Part model, mm, in its own coordinate system. Face numbers are marked on the shaded views. A direction names the side the tool comes from. Round coordinates to 2 decimals unless told otherwise and drop trailing zeros. Loops run counter-clockwise (first coordinate to the right, second up) from the corner with the lowest first, then second, coordinate; pieces in that order, holes last.
from build123d import *

# Parameters (mm, degrees)
BOSS_EXTRUDE1_DEPTH = 58
SKETCH2_R           = 6
BOSS_EXTRUDE2_DEPTH = 1
SKETCH3_R           = 4
BOSS_EXTRUDE3_DEPTH = 5
CUT_EXTRUDE1_DEPTH  = 3
FILLET1_R           = 0.5


with BuildPart() as part:
    # Sketch1 → Boss-Extrude1 (new body)
    with BuildSketch(Plane(origin=(0, 0, 0), x_dir=(1, 0, 0), z_dir=(0, 1, 0))):
        Polygon((0, 50), (0, 0), (50, 0), (50, 8), (30, 8), (8, 30), (8, 50), align=None)
        Polygon((5, 25.928932188), (25.928932188, 5), (5, 5), align=None, mode=Mode.SUBTRACT)
    extrude(amount=BOSS_EXTRUDE1_DEPTH)

    # Sketch2 → Boss-Extrude2 (add)
    with BuildSketch(Plane(origin=(8, 0, 0), x_dir=(0, 0, -1), z_dir=(1, 0, 0))):
        with Locations((40, 29)):
            Circle(SKETCH2_R)
    extrude(amount=BOSS_EXTRUDE2_DEPTH)

    # Sketch3 → Boss-Extrude3 (add)
    with BuildSketch(Plane(origin=(9, 0, 0), x_dir=(0, 0, -1), z_dir=(1, 0, 0))):
        with Locations((40, 29)):
            Circle(SKETCH3_R)
    extrude(amount=BOSS_EXTRUDE3_DEPTH)

    # Sketch4 → Cut-Extrude1 (cut)
    with BuildSketch(Plane(origin=(14, 0, 0), x_dir=(0, 0, -1), z_dir=(1, 0, 0))):
        Polygon((40, 26.401923789), (42.25, 27.700961894), (42.25, 30.299038106), (40, 31.598076211), (37.75, 30.299038106), (37.75, 27.700961894), align=None)
    extrude(amount=-CUT_EXTRUDE1_DEPTH, mode=Mode.SUBTRACT)

    # Fillet1
    fillet1_edges = [part.edges().sort_by_distance(p)[0] for p in [
        (14, 29, -36),
    ]]
    fillet(fillet1_edges, radius=FILLET1_R)


solid = part.part
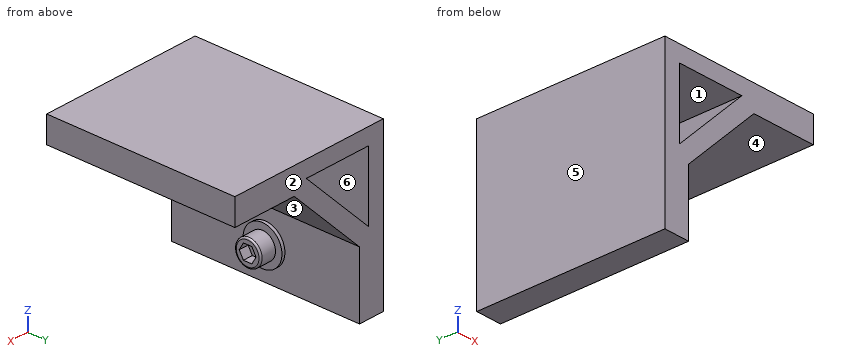
1) Slice it at B-B, the plane z = -7. Give the cut face in (x, y).
Values:
outline: (0, 0) - (5, 0) - (5, 58) - (0, 58) - close; (23.93, 0) - (50, 0) - (50, 58) - (23.93, 58) - close
2) Drop flat-ended pins along their axis: pin 1 Ø22 at (y, z) = (36, -35.5) entering from +X; pin 2 Ø2 at (y, z) = (30, -39.5) entering from +X; pin 3 Ø8 at (x, y) = (32.5, 12) entering from -Z. Give the stop position or say it passes through.
Values:
pin 1: stops at x = 14
pin 2: stops at x = 11
pin 3: stops at z = -9.5
3) Slice it at C-C, the plane x = 6. Give the cut face in (y, z).
Values:
outline: (0, -50) - (58, -50) - (58, -24.93) - (0, -24.93) - close; (0, -5) - (58, -5) - (58, 0) - (0, 0) - close
4) Mould opens along X. For the marked faces 1, 2 and 3 say: released by +X, released by -X, zero draft, split by the parting line, or undercut.
Values:
face 1: undercut
face 2: zero draft
face 3: released by +X
5) Tool access for the marked faces 4, 5 and 6: list every direction of +Z, -Z, +X, -X, +Y, -Y with a clear straight run to the whole face (end or side of a thin tool).
Values:
face 4: -Z, +X, +Y, -Y
face 5: +Z, -Z, -X, +Y, -Y
face 6: +Y, -Y
6) Slice it at D-D, the plane y = 17. Give the cut face in (x, z).
Values:
outline: (0, -50) - (8, -50) - (8, -30) - (30, -8) - (50, -8) - (50, 0) - (0, 0) - close; hole (5, -25.93) - (25.93, -5) - (5, -5) - close
7) Slice it at A-A, the plane y = 29. Give the cut face in (x, z), then the cut area to 3 significant figures.
Values:
outline: (0, -50) - (8, -50) - (8, -46) - (9, -46) - (9, -44) - (13.5, -44) arc R0.5 ccw to (14, -43.5) - (14, -42.25) - (11, -42.25) - (11, -37.75) - (14, -37.75) - (14, -36.5) arc R0.5 ccw to (13.5, -36) - (9, -36) - (9, -34) - (8, -34) - (8, -30) - (30, -8) - (50, -8) - (50, 0) - (0, 0) - close; hole (5, -25.93) - (25.93, -5) - (5, -5) - close
area: 797 mm2
8) Wall check: line 1 along Z through (x, y) = (22.5, 33); line 2 along X through (y, z) = (33, -25); line 3 along Z through (x, y) = (10, 52). Give the ranges that are in metal, low to high.
Values:
line 1: z = -15.5 to -8.43, -5 to 0
line 2: x = 0 to 5, 5.93 to 13
line 3: z = -28 to -20.93, -5 to 0
